For this review, take the finished solid that the model builds, in its own axes (mm). A direction names the side the tool comes from. Coordinates: 2 decimals unless noted, no trailing zeros. Write each loop counter-clockwise with the first axis right and the second up, starting at its lowest first coordinate (ties: lowest second). Pieces come first, ordered by that corner, then holes. Notation, with made-up numbers: M 3,2 L 20,2 A24 ccw 20,14 Z; hole C 82,-22 d8. An arc over 180 degrees is marked long. Return JSON: item names as keys, results as strings.
Autodesk Inventor part; units mm, degrees
ref_plane "YZ Plane" through (0, 0, 0) normal (1, 0, 0) x (0, 1, 0)
ref_plane "XY Plane" through (0, 0, 0) normal (0, 0, 1) x (1, 0, 0)
ref_plane "作業平面2" through (0, 6, 0) normal (0, 1, 0) x (-1, 0, 0)
sketch "スケッチ3" plane through (0, 6, 0) normal (0, 1, 0) x (-1, 0, 0)
  line L0 (3.975, -3.975) -> (-3.975, -3.975)
  line L1 (-3.975, -3.975) -> (-3.975, 3.975)
  line L2 (-3.975, 3.975) -> (3.975, 3.975)
  line L3 (3.975, 3.975) -> (3.975, -3.975)
  line L4 (3.975, -3.975) -> (-3.975, 3.975) construction
  line L5 (-3.975, -3.975) -> (3.975, 3.975) construction
  line L6 (5.025, -5.025) -> (-5.025, -5.025)
  line L7 (-5.025, -5.025) -> (-5.025, 5.025)
  line L8 (-5.025, 5.025) -> (5.025, 5.025)
  line L9 (5.025, 5.025) -> (5.025, -5.025)
  line L10 (5.025, -5.025) -> (-5.025, 5.025) construction
  line L11 (-5.025, -5.025) -> (5.025, 5.025) construction
  point P0 (0, 0)
  point P1 (0, 0)
  dimension "d19" = 7.95
  dimension "d20" = 7.95
  dimension "d21" = 10.05
  dimension "d22" = 10.05
sketch "スケッチ1" plane through (0, 0, 0) normal (0, 1, 0) x (-1, 0, 0)
  line L0 (6.5, -6.5) -> (-6.5, 6.5) construction
  line L1 (-6.5, -6.5) -> (6.5, 6.5) construction
  line L2 (1.046, 3.9037) -> (3.9037, 1.046)
  line L3 (3.9037, 1.046) -> (2.8577, -2.8577)
  line L4 (2.8577, -2.8577) -> (-1.046, -3.9037)
  line L5 (-1.046, -3.9037) -> (-3.9037, -1.046)
  line L6 (-3.9037, -1.046) -> (-2.8577, 2.8577)
  line L7 (-2.8577, 2.8577) -> (1.046, 3.9037)
  line L8 (-6.5, -6.5) -> (6.5, -6.5)
  line L9 (6.5, -6.5) -> (6.5, 6.5)
  line L10 (6.5, 6.5) -> (-6.5, 6.5)
  line L11 (-6.5, 6.5) -> (-6.5, -6.5)
  line L12 (-6.5, -6.5) -> (6.5, 6.5) construction
  line L13 (6.5, -6.5) -> (-6.5, 6.5) construction
  circle A0 centre (0, 0) radius 2.05
  dimension "d33" = 7
  dimension "d34" = 13
  dimension "d35" = 13
  dimension "d36" = 4.1
extrude "押し出し8" add sketch "スケッチ1" along normal blind 6 contours L2 L3 L4 L5 L6 L7 | L11 L10 L9 L8 | A0
extrude "押し出し9" cut sketch "スケッチ3" against normal blind 2
extrude "押し出し10" cut sketch "スケッチ1" along normal blind 3.2 contours L2 L3 L4 L5 L6 L7
extrude "押し出し11" cut sketch "スケッチ1" along normal blind 6 contours A0
properties part number "pin_joint_ver2_1"
1. Draft analysis for pull direction X (two halves, no side actions). For faces 4 (the face through (-6.5, 3, 0)), 5 (the face through (0, 3, -6.5)), 6 (the face through (3.388, 1.578, 0.879)), 7 (the face through (6.5, 3, 0)), state which applies: +X half, -X half, draft (parallel to the pull), parting line (faces both ways), or undercut.
Checks:
{"face 4": "-X half", "face 5": "draft", "face 6": "undercut", "face 7": "+X half"}
2. Clearance check with a flat-ended pin moving along its axis: pin 1 Ø4 at (x, z) = (0, -1.5) entering from -Y. State where the tip first meets the part, or that it passes through.
Checks:
{"pin 1": "y = 3.2"}
3. We need section B-B (z = 1.25). State the section outline as (x, y) points (3 decimals).
Checks:
{"outline": "M -6.5,0 L -3.7,0 L -3.7,3.2 L -1.625,3.2 L -1.625,6 L -3.975,6 L -3.975,4 L -5.025,4 L -5.025,6 L -6.5,6 Z; M 1.625,3.2 L 3.288,3.2 L 3.288,0 L 6.5,0 L 6.5,6 L 5.025,6 L 5.025,4 L 3.975,4 L 3.975,6 L 1.625,6 Z"}
4. For faces 1 (the face through (-2.455, 1.578, 2.495)), 2 (the face through (0, 3, 6.5)), 3 (the face through (3.975, 5, 0)), list the 3-axis set-ups (+Z, -Z, +X, -X, +Y, -Y) from which the entire face can be reached by the end or side of a thin tool; tool diameter is ignored.
Checks:
{"face 1": "-Y", "face 2": "+Z, +X, -X, +Y, -Y", "face 3": "+Y"}
5. Wall thickness on L1, parallel to Z at x = 0, y = 5.15 (3 decimals); L2, parallel to X at y = 4.95, z = 3.25 (3 decimals); L3, parallel to X at y = 4.6, z = 4.25 (3 decimals): over which ranges is each line inside the solid? List them lowest first. Write a range as from..to.
Checks:
{"L1": "-6.5..-5.025, -3.975..-2.05, 2.05..3.975, 5.025..6.5", "L2": "-6.5..-5.025, -3.975..3.975, 5.025..6.5", "L3": "-6.5..-5.025, 5.025..6.5"}
6. We need section C-C (x = 0). State the section outline as (y, z) points (3 decimals).
Checks:
{"outline": "M 0,-6.5 L 6,-6.5 L 6,-5.025 L 4,-5.025 L 4,-3.975 L 6,-3.975 L 6,-2.05 L 3.2,-2.05 L 3.2,-3.623 L 0,-3.623 Z; M 0,3.623 L 3.2,3.623 L 3.2,2.05 L 6,2.05 L 6,3.975 L 4,3.975 L 4,5.025 L 6,5.025 L 6,6.5 L 0,6.5 Z"}
7. We need section A-A (y = 4.45). State the section outline as (x, z) points (3 decimals).
Checks:
{"outline": "M -6.5,-6.5 L 6.5,-6.5 L 6.5,6.5 L -6.5,6.5 Z; M -3.975,-3.975 L 3.975,-3.975 L 3.975,3.975 L -3.975,3.975 Z; hole M -5.025,-5.025 L 5.025,-5.025 L 5.025,5.025 L -5.025,5.025 Z; hole C 0,0 d4.1"}
8. We need section D-D (y = 0.95). State the section outline as (x, z) points, plus the area to 3 significant figures.
Checks:
{"outline": "M -6.5,-6.5 L 6.5,-6.5 L 6.5,6.5 L -6.5,6.5 Z; hole M -3.9,1.05 L -2.86,-2.86 L 1.05,-3.9 L 3.9,-1.05 L 2.86,2.86 L -1.05,3.9 Z", "area": "127 mm2"}
